The model under review builds one solid part; all positions refer to its coordinate system, in mm. A direction names the side the tool comes from. Round coordinates to 2 decimals unless told otherwise and drop trailing zeros. Order: outer loops, then holes, each group sorted by start corner. A loop starts at its lowest first (then second) coordinate and runs counter-clockwise, first axis right, second up.
from build123d import *

# Parameters (mm, degrees)
BOSS_EXTRUDE1_DEPTH = 54
SKETCH7_W           = 12.542465984
SKETCH7_H           = 8.941456765
CUT_EXTRUDE4_DEPTH  = 4
SKETCH8_W           = 12.536281236
SKETCH8_H           = 9.084679825
CUT_EXTRUDE5_DEPTH  = 4
SKETCH10_R          = 50
CUT_EXTRUDE6_DEPTH  = 10
SKETCH12_W          = 173
SKETCH12_H          = 4
SKETCH12_H_2        = 4.470728383
BOSS_EXTRUDE2_DEPTH = 4


with BuildPart() as part:
    # Sketch1 → Boss-Extrude1 (new, symmetric)
    with BuildSketch(Plane(origin=(0, 0, 0), x_dir=(1, 0, 0), z_dir=(0, 1, 0))):
        Polygon((-63.408892702, 20.487993735), (122.091107298, 20.487993735), (122.091107298, 12.487993735), (118.091107298, 12.487993735), (118.091107298, 16.487993735), (113.591107298, 16.487993735), (113.591107298, 12.487993735), (109.591107298, 12.487993735), (109.591107298, 16.487993735), (-50.908892702, 16.487993735), (-50.908892702, 12.487993735), (-54.908892702, 12.487993735), (-54.908892702, 16.487993735), (-59.408892702, 16.487993735), (-59.408892702, 12.487993735), (-63.408892702, 12.487993735), align=None)
    extrude(amount=BOSS_EXTRUDE1_DEPTH, both=True)

    # Sketch7 → Cut-Extrude4 (cut)
    with BuildSketch(Plane.XY.offset(-12.487993735)):
        with Locations((115.819874306, 49.529271618)):
            Rectangle(SKETCH7_W, SKETCH7_H)
    extrude(amount=-CUT_EXTRUDE4_DEPTH, mode=Mode.SUBTRACT)

    # Sketch8 → Cut-Extrude5 (cut)
    with BuildSketch(Plane.XY.offset(-12.487993735)):
        with Locations((115.82296668, -49.457660088)):
            Rectangle(SKETCH8_W, SKETCH8_H)
    extrude(amount=-CUT_EXTRUDE5_DEPTH, mode=Mode.SUBTRACT)

    # Sketch10 → Cut-Extrude6 (cut)
    with BuildSketch(Plane.XY.offset(-12.487993735)):
        with Locations((-95.408892702, 0)):
            Circle(SKETCH10_R)
    extrude(amount=-CUT_EXTRUDE6_DEPTH, mode=Mode.SUBTRACT)

    # Sketch12 → Boss-Extrude2 (add)
    with BuildSketch(Plane.XY.offset(-16.487993735)):
        with Locations((35.591107298, -52)):
            Rectangle(SKETCH12_W, SKETCH12_H)
        with Locations((35.591107298, 51.764635809)):
            Rectangle(SKETCH12_W, SKETCH12_H_2)
    extrude(amount=BOSS_EXTRUDE2_DEPTH)


solid = part.part
(1) Clearance check with flat-ended pins moving along their axes: P1, Ø4.5, axis at y = -6.5, z = -14, coming from the -X side; P2, Ø1.3, axis at x = -57, y = 42, coming from the +Z side. State where each tip first meets the part, or that it passes through.
(2) We need section C-C (y = -41.5). Give the boundary of the cut face in (x, z).
(3) We need section A-A (z = -14.25). Give the boundary of the cut face in (x, y).
(4) We need section D-D (x = 40.5). Give the boundary of the cut face in (y, z), and give its area (3 significant figures).
(5) Tool access review of faces 4 (the flat face through (-63.409, 46, -16)), 5 (the flat face through (-54.909, 42, -14)), 6 (the flat face through (112, -44.915, -14)), 7 (the flat face through (-50.909, 36, -15)): name each direction out of +Z, -Z, +X, -X, +Y, -Y from which nothing blocks a thin tool from reaching the whole face with its end or side.
(6) To check wall thickness, follow L1, parallel to Y at x = -42.5, z = -13.75; L2, parallel to X at y = 39.5, z = -15.25; L3, parallel to X at y = -2.5, z = -15.75. State the ranges of each line that lie inside material, in increasing order.
(7) The part is to be moulded in two halves that separate along Y. For faces 1 (the flat face through (31, 54, -17)), 2 (the flat face through (-54.909, -41, -14)), 3 (the flat face through (37, 0, -16.488)), say which applies: pulls with the +Y half, pulls with the -Y half, needs draft (parallel to the pull), parting line crosses it, or undercut.
(8) We need section B-B (x = 111.5). Give the boundary of the cut face in (y, z), and give its area (3 significant figures).
Verdict:
1. P1: stops at x = 109.59
1. P2: stops at z = -16.49
2. outline: (-63.41, -20.49) - (122.09, -20.49) - (122.09, -12.49) - (118.09, -12.49) - (118.09, -16.49) - (113.59, -16.49) - (113.59, -12.49) - (109.59, -12.49) - (109.59, -16.49) - (-50.91, -16.49) - (-50.91, -12.49) - (-54.91, -12.49) - (-54.91, -16.49) - (-59.41, -16.49) - (-59.41, -12.49) - (-63.41, -12.49) - close
3. outline: (-63.41, -54) - (-59.41, -54) - (-59.41, -34.7) arc R50 cw to (-63.41, -38.42) - close; (-63.41, 38.42) arc R50 cw to (-59.41, 34.7) - (-59.41, 54) - (-63.41, 54) - close; (-54.91, -54) - (122.09, -54) - (122.09, -50) - (-50.91, -50) - (-50.91, -22.8) arc R50 cw to (-54.91, -29.32) - close; (-54.91, 29.32) arc R50 cw to (-50.91, 22.8) - (-50.91, 49.53) - (122.09, 49.53) - (122.09, 54) - (-54.91, 54) - close; (109.59, -44.92) - (113.59, -44.92) - (113.59, 45.06) - (109.59, 45.06) - close; (118.09, -44.92) - (122.09, -44.92) - (122.09, 45.06) - (118.09, 45.06) - close
4. outline: (-54, -20.49) - (54, -20.49) - (54, -12.49) - (49.53, -12.49) - (49.53, -16.49) - (-50, -16.49) - (-50, -12.49) - (-54, -12.49) - close
4. area: 466 mm2
5. face 4: +Z, -Z, -X, +Y, -Y
5. face 5: +Z, +Y, -Y
5. face 6: +Z, +X
5. face 7: +Z
6. L1: y = -54 to -50, 49.53 to 54
6. L2: x = -63.41 to -59.41, -54.91 to -50.91, 109.59 to 113.59, 118.09 to 122.09
6. L3: x = 109.59 to 113.59, 118.09 to 122.09
7. face 1: pulls with the +Y half
7. face 2: needs draft
7. face 3: undercut
8. outline: (-54, -20.49) - (54, -20.49) - (54, -12.49) - (49.53, -12.49) - (49.53, -16.49) - (45.06, -16.49) - (45.06, -12.49) - (-44.92, -12.49) - (-44.92, -16.49) - (-50, -16.49) - (-50, -12.49) - (-54, -12.49) - close
8. area: 826 mm2
